Autodesk Inventor part; units mm, degrees
ref_plane "YZ Plane" through (0, 0, 0) normal (1, 0, 0) x (0, 1, 0)
ref_plane "XZ Plane" through (0, 0, 0) normal (0, 1, 0) x (-1, 0, 0)
ref_plane "XY Plane" through (0, 0, 0) normal (0, 0, 1) x (1, 0, 0)
sketch "Sketch2" plane through (0, 0, 0) normal (0, 0, 1) x (1, 0, 0)
  circle A0 centre (-32, 0) radius 7.5 construction
  circle A1 centre (32, 0) radius 7.5 construction
  circle A2 centre (0, 0) radius 5
  line L0 (-13.5, 14) -> (13.5, 14)
  line L1 (13.5, 14) -> (13.5, 11)
  line L2 (13.5, 11) -> (25.5, 11)
  line L3 (25.5, 11) -> (25.5, 14)
  line L4 (25.5, 14) -> (37, 14)
  line L5 (37, 14) -> (37, 11)
  line L6 (37, 11) -> (40, 11)
  line L7 (40, 11) -> (40, 8)
  line L8 (40, 8) -> (43, 8)
  line L9 (43, 8) -> (43, -8)
  line L10 (43, -8) -> (40, -8)
  line L11 (40, -8) -> (40, -11)
  line L12 (40, -11) -> (37, -11)
  line L13 (37, -11) -> (37, -14)
  line L14 (37, -14) -> (25.5, -14)
  line L15 (25.5, -14) -> (25.5, -11)
  line L16 (25.5, -11) -> (13.5, -11)
  line L17 (13.5, -11) -> (13.5, -14)
  line L18 (13.5, -14) -> (-13.5, -14)
  line L19 (-13.5, -14) -> (-13.5, -11)
  line L20 (-13.5, -11) -> (-25.5, -11)
  line L21 (-25.5, -11) -> (-25.5, -14)
  line L22 (-25.5, -14) -> (-37, -14)
  line L23 (-37, -14) -> (-37, -11)
  line L24 (-37, -11) -> (-40, -11)
  line L25 (-40, -11) -> (-40, -8)
  line L26 (-40, -8) -> (-43, -8)
  line L27 (-43, -8) -> (-43, 8)
  line L28 (-43, 8) -> (-40, 8)
  line L29 (-40, 8) -> (-40, 11)
  line L30 (-40, 11) -> (-37, 11)
  line L31 (-37, 11) -> (-37, 14)
  line L32 (-37, 14) -> (-25.5, 14)
  line L33 (-25.5, 14) -> (-25.5, 11)
  line L34 (-25.5, 11) -> (-13.5, 11)
  line L35 (-13.5, 11) -> (-13.5, 14)
  circle A3 centre (-32, 0) radius 6
  circle A4 centre (32, 0) radius 6
  line L36 (25.5, 11) -> (-25.5, 11)
  line L37 (-25.5, 14) -> (-25.5, 11)
  line L38 (-25.5, 14) -> (-37, 14)
  line L39 (-37, 11) -> (-37, 14)
  line L40 (-37, 11) -> (-40, 11)
  line L41 (-40, 8) -> (-40, 11)
  line L42 (-40.3391, 8) -> (-43, 8)
  line L43 (-43, -8) -> (-43, 8)
  line L44 (-43, -8) -> (-40, -8)
  line L45 (-40, -11) -> (-40, -8)
  line L46 (-40, -11) -> (-37, -11)
  line L47 (-37, -11) -> (-37, -14)
  line L48 (-37, -14) -> (-25.5, -14)
  line L49 (-25.5, -11) -> (-25.5, -14)
  line L50 (-25.5, -11) -> (-13.5, -11)
  line L51 (-13.5, -11) -> (-13.5, -14)
  line L52 (13.5, -14) -> (-13.5, -14)
  line L53 (13.5, -11) -> (13.5, -14)
  line L54 (13.5, -11) -> (25.5, -11)
  line L55 (25.5, -11) -> (25.5, -14)
  line L56 (25.5, -14) -> (37, -14)
  line L57 (37, -11) -> (37, -14)
  line L58 (37, -11) -> (40, -11)
  line L59 (40, -11) -> (40, -8)
  line L60 (40, -8) -> (43, -8)
  line L61 (43, -8) -> (43, 8)
  line L62 (43, 8) -> (40, 8)
  line L63 (40, 8) -> (40, 11)
  line L64 (37, 11) -> (40, 11)
  line L65 (37, 11) -> (37, 14)
  line L66 (37, 14) -> (25.5, 14)
  line L67 (25.5, 14) -> (25.5, 11)
  dimension "d11" = 12
  dimension "d12" = 12
extrude "Extrusion1" add sketch "Sketch2" along normal blind 3 contours L36 L2 L3 L4 L5 L6 L7 L8 L9 L10 L11 L12 L13 L14 L15 L16 L17 L18 L19 L20 L21 L22 L23 L24 L25 L26 L27 L28 L29 L30 L31 L32 L33 L34
properties part number "Bearing-Outer"
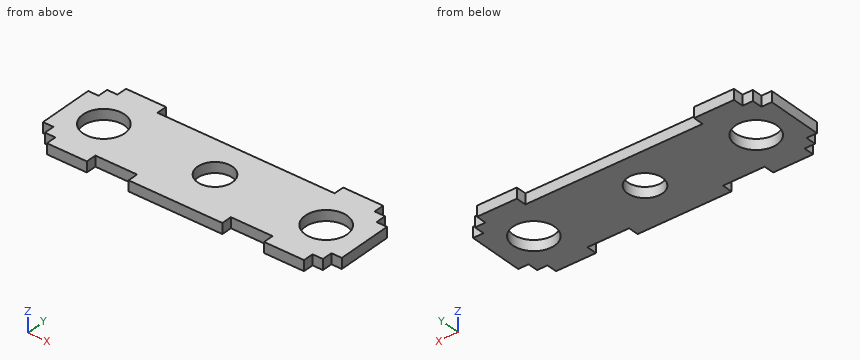
Check sheet for the modelled part. Datum: model origin and axes. Units: mm. Coordinates: 2 decimals unless noted, no trailing zeros. Order: outer loops, then holes, each group sorted by start corner. A loop starts at its lowest first (then second) coordinate and runs counter-clockwise, first axis right, second up. Notation, with made-up numbers: M -6.5,57.25 L 40.5,57.25 A19 cw 40.5,81.25 Z; hole C 31.25,58.5 d9. An arc over 180 degrees is marked long. One line per question, with ' | ' between items. Start each with the question number.
Item 1: Sectioned sample at A-A on y = 0. Record the cut outline in (x, z).
Item 2: Sectioned sample at B-B on x = 0. Record the cut outline in (y, z).
Item 3: Sectioned sample at C-C on x = -32. Record the cut outline in (y, z).
Item 4: Material ranges on line 1 (Y direction, x = -32, z = 1.85); line 2 (X direction, y = -2.75, z = 2.5); line 3 (X direction, y = 11.5, z = 0.6), recorded low to high.
Item 5: Gauge pin test, flat ends, axial feed: P1, Ø0.9, axis at y = -12, z = 1, coming from the +X side; P2, Ø1.5, axis at y = 9.5, z = 1, coming from the +X side; P3, Ø0.9, axis at x = -39, z = 1.5, coming from the -Y side. Record the tip position at first contact, or that the pin passes through.
Item 6: Sectioned sample at D-D on z = 0.65. Count the separate pieces of the cut face and the enclosed holes in it, and give its area (3 significant figures).
Answer below:
1) outline: M -43,0 L -38,0 L -38,3 L -43,3 Z; M -26,0 L -5,0 L -5,3 L -26,3 Z; M 5,0 L 26,0 L 26,3 L 5,3 Z; M 38,0 L 43,0 L 43,3 L 38,3 Z
2) outline: M -14,0 L -5,0 L -5,3 L -14,3 Z; M 5,0 L 11,0 L 11,3 L 5,3 Z
3) outline: M -14,0 L -6,0 L -6,3 L -14,3 Z; M 6,0 L 14,0 L 14,3 L 6,3 Z
4) line 1: y = -14 to -6, 6 to 14 | line 2: x = -43 to -37.33, -26.67 to -4.18, 4.18 to 26.67, 37.33 to 43 | line 3: x = -37 to -25.5, 25.5 to 37
5) P1: stops at x = 37 | P2: stops at x = 40 | P3: stops at y = -11
6) separate pieces: 1 | enclosed holes: 3 | area: 1,770 mm^2
